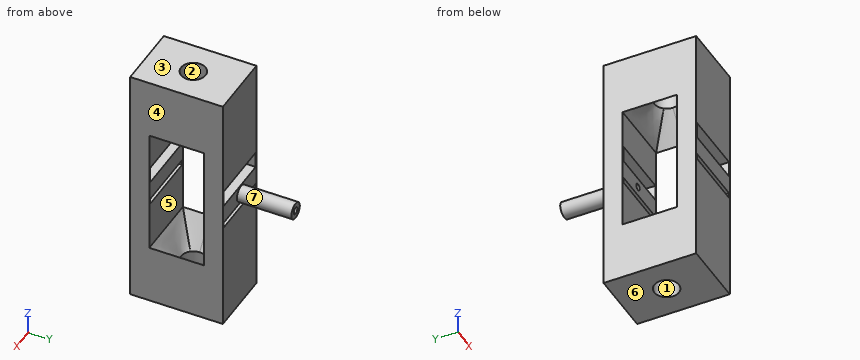
Autodesk Inventor part; units mm, degrees
ref_plane "YZ Plane" through (0, 0, 0) normal (1, 0, 0) x (0, 1, 0)
ref_plane "XZ Plane" through (0, 0, 0) normal (0, 1, 0) x (-1, 0, 0)
ref_plane "XY Plane" through (0, 0, 0) normal (0, 0, 1) x (1, 0, 0)
sketch "Sketch1" plane through (0, 0, 0) normal (0, 1, 0) x (-1, 0, 0)
  line L0 (0, 0) -> (-24, 0)
  line L1 (-24, 0) -> (-24, -91)
  line L2 (-24, -91) -> (0, -91)
  line L3 (0, -91) -> (0, 0)
  dimension "d0" = 91
  dimension "d1" = 24
extrude "Extrusion1" add sketch "Sketch1" along normal blind 34
sketch "Sketch2" plane through (24, 0, 0) normal (1, 0, 0) x (0, 0, -1)
  line L0 (22, 27) -> (69, 27)
  line L1 (69, 27) -> (69, 7)
  line L2 (69, 7) -> (22, 7)
  line L3 (22, 7) -> (22, 27)
  line L4 (0, 34) -> (91, 34)
  line L5 (0, 0) -> (91, 0)
  line L6 (0, 0) -> (0, 34)
  line L7 (91, 0) -> (91, 34)
  dimension "d4" = 7
  dimension "d5" = 7
  dimension "d6" = 22
  dimension "d7" = 22
extrude "Extrusion2" cut sketch "Sketch2" against normal up to surface (24 mm away) contours L0 L1 L2 L3
sketch "Sketch3" plane through (0, 34, 0) normal (0, 1, 0) x (1, 0, 0)
  line L0 (0.5, 42) -> (23.5, 42)
  line L1 (23.5, 42) -> (23.5, 36)
  line L2 (23.5, 36) -> (0.5, 36)
  line L3 (0.5, 36) -> (0.5, 42)
  line L4 (0, 91) -> (0, 0)
  line L5 (24, 0) -> (24, 91)
  line L6 (0, 0) -> (24, 0)
  dimension "d10" = 0.5
  dimension "d11" = 0.5
  dimension "d12" = 6
  dimension "d13" = 36
extrude "Extrusion3" cut sketch "Sketch3" against normal up to surface (34 mm away)
sketch "Sketch4" plane through (0, 34, 0) normal (0, 1, 0) x (1, 0, 0)
  line L0 (0.5, 51) -> (23.5, 51)
  line L1 (23.5, 51) -> (23.5, 49)
  line L2 (23.5, 49) -> (0.5, 49)
  line L3 (0.5, 49) -> (0.5, 51)
  line L4 (0.5, 42) -> (23.5, 42)
  line L5 (24, 0) -> (24, 91)
  line L6 (0, 91) -> (0, 0)
  dimension "d16" = 2
  dimension "d17" = 7
  dimension "d18" = 0.5
  dimension "d19" = 0.5
extrude "Extrusion4" cut sketch "Sketch4" against normal up to surface (34 mm away)
sketch "Sketch5" plane through (0, 0, 0) normal (0, 0, 1) x (1, 0, 0)
  circle A0 centre (12, 17) radius 4.5
  line L0 (0, 0) -> (24, 0)
  line L1 (24, 0) -> (24, 34)
  dimension "d22" = 17
  dimension "d23" = 12
  dimension "d24" = 9
extrude "Extrusion5" cut sketch "Sketch5" against normal blind 12
loft "Loft1" cut section 1 edges at (7.5, 17, -12) section 2 edges at (0, 17, -22) (12, 27, -22) (24, 17, -22) (12, 7, -22)
sketch "Sketch6" plane through (24, 0, -91) normal (0, 0, -1) x (-1, 0, 0)
  circle A0 centre (12, 17) radius 4.5
  line L0 (24, 0) -> (24, 34)
  line L1 (0, 0) -> (24, 0)
  dimension "d31" = 12
  dimension "d32" = 17
  dimension "d33" = 9
extrude "Extrusion6" cut sketch "Sketch6" against normal blind 12
loft "Loft2" cut section 1 edges at (16.5, 17, -79) section 2 edges at (0, 17, -69) (12, 7, -69) (24, 17, -69) (12, 27, -69)
sketch "Sketch7" plane through (0, 34, 0) normal (0, 1, 0) x (1, 0, 0)
  circle A0 centre (11, 45.5) radius 3
  line L0 (0, 91) -> (0, 0)
  line L1 (24, 0) -> (24, 91)
  line L2 (0.5, 42) -> (23.5, 42)
  line L3 (23.5, 49) -> (0.5, 49)
  dimension "d40" = 11
  dimension "d41" = 13
  dimension "d42" = 3.5
  dimension "d43" = 3.5
  dimension "d44" = 6
extrude "Extrusion7" add sketch "Sketch7" along normal blind 20
sketch "Sketch8" plane through (11, 54, -45.5) normal (0, 1, 0) x (1, 0, 0)
  circle A0 centre (0, 0) radius 1.25
  point P0 (-11, -45.5)
  dimension "d47" = 2.5
extrude "Extrusion8" cut sketch "Sketch8" against normal up to surface (27 mm away)
properties part number "20220727_1cell_PBME"
The model under review builds one solid part; all positions refer to its coordinate system, in mm. Face numbers are marked on the shaded views. A direction names the side the tool comes from. Coordinates: 2 decimals unless noted, no trailing zeros. Order: outer loops, then holes, each group sorted by start corner. A loop starts at its lowest first (then second) coordinate and runs counter-clockwise, first axis right, second up. Notation, with made-up numbers: M -8.5,-24.75 L 28.5,-24.75 A32 cw 28.5,6.25 Z; hole C -19,23.25 d6. An arc over 180 degrees is marked long. One line per question, with ' | ' between items.
(1) Add section B-B, the plane z = -67. Write out the cut boundary in (x, y), then the cut area to 3 significant figures.
Geometry results:
outline: M 0,0 L 24,0 L 24,7 L 0,7 Z; M 0,27 L 24,27 L 24,34 L 0,34 Z | area: 336 mm²
(2) Add section D-D, the plane x = 4. State how many separate pieces and enclosed holes the cut face has, then the cut area to 3 significant figures.
Geometry results:
separate pieces: 4 | enclosed holes: 0 | area: 1,870 mm²
(3) The part is to be moulded in two halves that separate along X. For the marked faces 1, 2, 3 and 4, say which applies: +X half, -X half, draft (parallel to the pull), parting line (faces both ways), or undercut.
Geometry results:
face 1: undercut | face 2: undercut | face 3: draft | face 4: +X half
(4) Machinability: for the marked faces 5, 6 and 7, which of the approach directions +Z, -Z, +X, -X, +Y, -Y give a long, thin tool a straight path to every point of the face, cutting with its end or side? Answer none if there is none.
Geometry results:
face 5: +X, -X | face 6: -Z, +X, -X, +Y, -Y | face 7: +Y
(5) Add section C-C, the plane y = 38. Write out the cut boundary in (x, z).
Geometry results:
outline: C 11,-45.5 d6; hole C 11,-45.5 d2.5
(6) For probe 1 along Z at (x, y) = (5, 29); probe 2 along X at (y, z) = (17, -8); probe 3 along Y at (x, z) = (12, -4.25), list the stretches that pass through material, from the lowest coordinate up. Write a range as from..to.
Geometry results:
probe 1: z = -91..-51, -49..-42, -36..0 | probe 2: x = 0..7.5, 16.5..24 | probe 3: y = 0..12.5, 21.5..34
(7) Insertion check: pin 1 (1.5 mm diameter, centred on y = 36, z = -76, fed in from +X); pin 2 (1.5 mm diameter, centred on x = 11, z = -45.5, fed in from +Y); pin 3 (2 mm diameter, centred on x = 8, y = 40, fed in from +Z). Each pin has a flat end and moves straight along its axis. Give the tip position at first contact, or say it passes through.
Geometry results:
pin 1: passes through | pin 2: stops at y = 7 | pin 3: stops at z = -43.26
(8) Add section A-A, the plane z = -40. Write out the cut boundary in (x, y), then the cut area to 3 significant figures.
Geometry results:
outline: M 0,0 L 0.5,0 L 0.5,7 L 0,7 Z; M 0,27 L 0.5,27 L 0.5,34 L 0,34 Z; M 23.5,0 L 24,0 L 24,7 L 23.5,7 Z; M 23.5,27 L 24,27 L 24,34 L 23.5,34 Z | area: 14.0 mm²
